Read the model definition and answer for the solid it produces. Units are mm, in the model's axes. A direction names the side the tool comes from. Coordinates: 2 decimals unless noted, no trailing zeros. Write each loop counter-clockwise with the first axis right and the second up, starting at its lowest first coordinate (ties: lowest second). Pieces come first, ordered by that corner, then holes. Notation, with made-up numbers: (38.25, -29.75) - (85.25, -29.75) arc R21 cw to (85.25, -3.75) - close; hole circle Ø6 at (-7, 66). An arc over 180 degrees is marked (long way). Use a Markdown table: item, result.
from build123d import *

# Parameters (mm, degrees)
F2_R     = 2.5
F3_DEPTH = 31.392483
F5_DEPTH = 12.5
F7_DEPTH = 12.5


with BuildPart() as f1:
    # F0 (on Front) → F1 (revolve)
    with BuildSketch(Plane.XZ):
        with BuildLine():
            ThreePointArc((3.844224, -8.787564), (3.659325, -7.666848), (4.312913, -6.737862))
            ThreePointArc((4.312913, -6.737862), (7.893777, -1.299338), (6.244998, 5))
            Line((6.244998, 5), (0, 5))
            Line((0, 5), (0, -8))
            Line((0, -8), (0, -12.891483))
            ThreePointArc((0, -12.891483), (7.462406, -17.623671), (6.363961, -26.391483))
            Line((6.363961, -26.391483), (8.215838, -26.391483))
            ThreePointArc((8.215838, -26.391483), (9.749656, -21.223349), (8.302841, -16.030187))
            Line((8.302841, -16.030187), (3.844224, -8.787564))
        make_face()
    revolve(axis=Axis((0, 0, -19.641483), (0, 0, -1)))

    # F2 (on face) → F3 (cut, through all)
    with BuildSketch(Plane.XY.offset(5)):
        Circle(F2_R)
    extrude(amount=-F3_DEPTH, mode=Mode.SUBTRACT)

    # F4 (on Front) → F5 (cut, symmetric)
    with BuildSketch(Plane.XZ):
        with BuildLine():
            Line((-1.5, -20.391483), (-1.5, -26.391483))
            Line((-1.5, -26.391483), (1.5, -26.391483))
            Line((1.5, -26.391483), (1.5, -20.391483))
            ThreePointArc((1.5, -20.391483), (0, -18.891483), (-1.5, -20.391483))
        make_face()
    extrude(amount=F5_DEPTH, both=True, mode=Mode.SUBTRACT)

    # F6 (on Right) → F7 (cut, symmetric)
    with BuildSketch(Plane.YZ):
        with BuildLine():
            Line((-1.5, -20.391483), (-1.5, -26.391483))
            Line((-1.5, -26.391483), (1.5, -26.391483))
            Line((1.5, -26.391483), (1.5, -20.391483))
            ThreePointArc((1.5, -20.391483), (0, -18.891483), (-1.5, -20.391483))
        make_face()
    extrude(amount=F7_DEPTH, both=True, mode=Mode.SUBTRACT)


solid = f1.part
(1) For faces 1 (the flat face through (-5, -5, -26.391)), 2 (the flat face through (1.5, -8.3, -23.4)), 3 (the flat face through (8.3, 1.5, -23.4)), determine the directions among +Z, -Z, +X, -X, +Y, -Y from which every point of the face is accessible in a straight line to the end or side of a thin tool.
Report:
| item | result |
|---|---|
| face 1 | -Z, +X, -X, +Y, -Y |
| face 2 | -Z, +Y, -Y |
| face 3 | -Z, +X, -X |
(2) A cutting plane is placed at B-B, the plane z = -12.5. Write down the section's boundary in (x, y).
Report:
| item | result |
|---|---|
| outline | circle Ø12.26 at (0, 0); hole circle Ø5 at (0, 0) |
(3) Straight lines are drawn through the part: L1, parallel to X at y = 0, z = 1; L2, parallel to Z at x = 4.75, y = 5.5; L3, parallel to X at y = 0, z = -7.5. For each, find the intervals that lie inside material, in ascending order.
Report:
| item | result |
|---|---|
| L1 | x = -7.94 to -2.5, 2.5 to 7.94 |
| L2 | z = -26.39 to -25.05, -17.24 to -14.35, -3.34 to 3.34 |
| L3 | x = -3.71 to -2.5, 2.5 to 3.71 |
(4) A cutting plane is placed at A-A, the plane z = -19.5. Count the separate pieces of the cut face and the enclosed holes in it, and give its area (3 significant figures).
Report:
| item | result |
|---|---|
| separate pieces | 4 |
| enclosed holes | 0 |
| area | 70.1 mm² |
(5) The mould has two halves that part along Z. Classify faces 4 (the flat face through (5, 5, -26.391)), 5 (the conical face through (-0.988, 4.448, -9.944)), 6 (the flat face through (1.5, 8.3, -23.4)): pulls with the +Z half, pulls with the -Z half, needs draft (parallel to the pull), parting line crosses it, or undercut.
Report:
| item | result |
|---|---|
| face 4 | pulls with the -Z half |
| face 5 | undercut |
| face 6 | needs draft |
(6) Each of these flat-tipped pins is pushed along its axis until it touches: P1, Ø1.7, axis at x = -8.5, z = -25, coming from the +Y side; P2, Ø3, axis at x = 8.5, z = -24.5, coming from the +Y side; P3, Ø1, axis at y = 7, z = -22.5, coming from the +X side. Where does it stop, or does it pass through?
Report:
| item | result |
|---|---|
| P1 | stops at y = 4.8 |
| P2 | stops at y = 6.06 |
| P3 | stops at x = 7.15 |
